```python
from build123d import *

# Parameters (mm, degrees)
EXTRUDE1_DEPTH     = 2.413
SKETCH2_R          = 1.1811
EXTRUDE2_DEPTH     = 1.524
SKETCH3_W          = 3.103966911
SKETCH3_H          = 0.635
CUT_EXTRUDE1_DEPTH = 0.7874
SKETCH4_R          = 0.254
EXTRUDE3_DEPTH     = 5.588


with BuildPart() as part:
    # Sketch1 → Extrude1 (new, symmetric)
    with BuildSketch(Plane(origin=(0, 0, 0), x_dir=(0, 0, -1), z_dir=(1, 0, 0))):
        Polygon((-9.525, 3.175), (9.525, 3.175), (9.525, -3.175), (8.763, -3.175), (8.763, -2.794), (-8.763, -2.794), (-8.763, -3.175), (-9.525, -3.175), align=None)
    extrude(amount=EXTRUDE1_DEPTH, both=True)

    # Sketch2 → Extrude2 (add)
    with BuildSketch(Plane.XY.offset(9.525)):
        with Locations(Location((0, 1.524, 0), (0, 0, 180))):
            Circle(SKETCH2_R)
    extrude(amount=EXTRUDE2_DEPTH)

    # Sketch3 → Cut-Extrude1 (cut)
    with BuildSketch(Plane.XY.offset(11.049)):
        with Locations((-0.005969167, 1.524)):
            Rectangle(SKETCH3_W, SKETCH3_H)
    extrude(amount=-CUT_EXTRUDE1_DEPTH, mode=Mode.SUBTRACT)

    # Sketch4 → Extrude3 (add)
    with BuildSketch(Plane.XZ.offset(2.794)):
        with Locations(Location((1.016, 6.223, 0), (0, 0, 90))):
            Circle(SKETCH4_R)
        with Locations(Location((-1.524, 1.143, 0), (0, 0, 90))):
            Circle(SKETCH4_R)
        with Locations(Location((1.016, -6.477, 0), (0, 0, 90))):
            Circle(SKETCH4_R)
    extrude(amount=EXTRUDE3_DEPTH)


solid = part.part
```
CAD build for the part. Positions are in the model's coordinates, mm. A direction names the side the tool comes from. Round coordinates to 2 decimals unless told otherwise and drop trailing zeros. Loops run counter-clockwise (first coordinate to the right, second up) from the corner with the lowest first, then second, coordinate; pieces in that order, holes last. Notation, with made-up numbers: M 66.5,0.5 L 96.5,0.5 A24 ccw 96.5,34.5 Z; hole C 17.5,-12 d11. An arc over 180 degrees is marked long. Use a Markdown table: item, result. Add a question column.
(1) Cut at D-D (z = 3.25). Give the cut face in (x, y) (3 decimals).
(2) Cut at B-B (y = 1). Give the cut face in (x, z) (1 decimal).
(3) Flat gauge pins, fed straight in: pin 1 (1.5 mm diameter, centred on y = -4, z = -6.5, fed in from -X); pin 2 (0.6 mm diameter, centred on x = 0.5, z = 9, fed in from -Y) (3 decimals); pin 3 (2.5 mm diameter, centred on x = 0.5, y = -1, fed in from +Z) (3 decimals). Where does each tip first touch, or does it go through?
(4) Which spindle directions (+Z, -Z, +X, -X, +Y, -Y) get a long thin tool onto all of the face, cutting with end or side? Do faces 1 (the face through (-1.127, 1.169, 10.107)), 2 (the face through (0, 3.175, 0)). Say none if no direction does.
(5) Cut at C-C (y = -6.75). Give the cut face in (x, z).
(6) Drill centre lines: line 1 (Z direction, x = -1.7, y = -1) (3 decimals); line 2 (Y direction, x = -2, z = 7.75) (3 decimals); line 3 (Z direction, x = 1.2, y = -3.25). Where is each one in solid material? Low to high.
(7) Pull direction Z, two halves, no side cores. Call faces 3 (the face through (0, -2.794, 0)), 4 (the face through (2.413, 0, 0)), 5 (the face through (0, 0, -9.525)), 6 (the face through (0, 1, 11.049)): +Z half, -Z half, draft (parallel to the pull), parting line (faces both ways), or undercut.
Geometry says:
| question | item | result |
|---|---|---|
| 1 | outline | M -2.413,-2.794 L 2.413,-2.794 L 2.413,3.175 L -2.413,3.175 Z |
| 2 | outline | M -2.4,-9.5 L 2.4,-9.5 L 2.4,9.5 L 1.1,9.5 L 1.1,11 L -1.1,11 L -1.1,9.5 L -2.4,9.5 Z |
| 3 | pin 1 | stops at x = 0.76 |
| 3 | pin 2 | stops at y = -3.175 |
| 3 | pin 3 | stops at z = 9.525 |
| 4 | face 1 | +Z |
| 4 | face 2 | +Z, -Z, +X, -X, +Y |
| 5 | outline | C -1.52,1.14 d0.51; C 1.02,-6.48 d0.51; C 1.02,6.22 d0.51 |
| 6 | line 1 | z = -9.525 to 9.525 |
| 6 | line 2 | y = -2.794 to 3.175 |
| 6 | line 3 | z = -6.65 to -6.3, 6.05 to 6.4 |
| 7 | face 3 | undercut |
| 7 | face 4 | draft |
| 7 | face 5 | -Z half |
| 7 | face 6 | +Z half |
